Geometry check sheet. Reference: the model listing, model coordinates, mm. A direction names the side the tool comes from. Give positions to 0.01 mm unless a question says otherwise; leave off trailing zeros. Loops run counter-clockwise (first coordinate to the right, second up) from the corner with the lowest first, then second, coordinate; pieces in that order, holes last. Notation, with made-up numbers: (67.5, -9) -> (115.5, -9) arc R32 cw to (115.5, 22) -> close; hole circle Ø5 at (78.5, 77). An arc over 180 degrees is marked (long way). Answer as a JSON object with one key per item and string values.
from build123d import *

# Parameters (mm, degrees)
F1_DEPTH = 50.8
F2_W     = 38.1
F2_H     = 25.4
F3_DEPTH = 38.101
F5_D     = 12.7


with BuildPart() as f1:
    # F0 (on Front) → F1 (new body)
    with BuildSketch(Plane.XZ):
        Polygon((-41.500658, 3.663934), (-60.550658, 3.663934), (-60.550658, -34.436066), (28.349342, -34.436066), (28.349342, 3.663934), (15.649342, 3.663934), (15.649342, -17.219239), (-41.500658, -17.219239), align=None)
    extrude(amount=F1_DEPTH)

    # F2 (on face) → F3 (cut, through all)
    with BuildSketch(Plane(origin=(0, 0, -34.436066), x_dir=(1, 0, 0), z_dir=(0, 0, -1))):
        with Locations((9.299342, 38.1)):
            Rectangle(F2_W, F2_H)
    extrude(amount=-F3_DEPTH, mode=Mode.SUBTRACT)

    # F5 (through all)
    with Locations(Plane.XY.offset(-17.219239)):
        with Locations((-28.852955, -40.337186), (0, -9.016548)):
            Hole(F5_D / 2)


solid = f1.part
1) Depth check by flat-ended pin: P1, Ø10, axis at y = -36.5, z = -12, coming from the +X side; P2, Ø6, axis at x = -31.5, z = -12, coming from the -Y side; P3, Ø14.5, axis at x = -28.85, y = -40.34, coming from the +Z side; P4, Ø5, axis at y = -34, z = -25.5, coming from the +X side. Enter the tip coordinate at first touch or a pass-through.
Geometry check:
{"P1": "stops at x = -41.5", "P2": "passes through", "P3": "stops at z = -17.22", "P4": "stops at x = -9.75"}
2) Tool access check on faces 1 (the face through (-19, -19, -17.219)), 2 (the face through (28.349, -13, -16)), 3 (the face through (13, -25.4, -20)). Record the directions out of +Z, -Z, +X, -X, +Y, -Y that give a thin tool (end or side, any length) a straight path to the whole face; none if there is none.
Geometry check:
{"face 1": "+Z, +Y, -Y", "face 2": "+Z, -Z, +X, +Y, -Y", "face 3": "+Z, -Z, +X, -Y"}
3) Section check B-B on x = 0. Record the cut outline in (y, z).
Geometry check:
{"outline": "(-25.4, -34.44) -> (-15.37, -34.44) -> (-15.37, -17.22) -> (-25.4, -17.22) -> close; (-2.67, -34.44) -> (0, -34.44) -> (0, -17.22) -> (-2.67, -17.22) -> close"}
4) Material ranges on line 1 along X through (y, z) = (-16, -11.5); line 2 along Y through (x, z) = (0, -26.75); line 3 along Z through (x, y) = (-38, -17), recorded low to high. Write a range as from..to.
Geometry check:
{"line 1": "x = -60.55..-41.5, 15.65..28.35", "line 2": "y = -25.4..-15.37, -2.67..0", "line 3": "z = -34.44..-17.22"}
5) Section check D-D on y = -21.5. Record the cut outline in (x, z).
Geometry check:
{"outline": "(-60.55, -34.44) -> (28.35, -34.44) -> (28.35, 3.66) -> (15.65, 3.66) -> (15.65, -17.22) -> (-41.5, -17.22) -> (-41.5, 3.66) -> (-60.55, 3.66) -> close"}
6) Section check A-A on z = -1. Record the cut outline in (x, y), plus the area to 3 significant figures.
Geometry check:
{"outline": "(-60.55, -50.8) -> (-41.5, -50.8) -> (-41.5, 0) -> (-60.55, 0) -> close; (15.65, -25.4) -> (28.35, -25.4) -> (28.35, 0) -> (15.65, 0) -> close", "area": "1,290 mm2"}
7) Draft check along X on faces 4 (the face through (-51, -25, 3.664)), 5 (the face through (-9.751, -38, -26)), 6 (the face through (15.649, -13, -7)). Enter one of: pulls with the +X half, pulls with the -X half, needs draft (parallel to the pull), parting line crosses it, or undercut.
Geometry check:
{"face 4": "needs draft", "face 5": "pulls with the +X half", "face 6": "undercut"}
8) Section check C-C on z = -23.5. Record the cut outline in (x, y).
Geometry check:
{"outline": "(-60.55, -50.8) -> (-9.75, -50.8) -> (-9.75, -25.4) -> (28.35, -25.4) -> (28.35, 0) -> (-60.55, 0) -> close; hole circle Ø12.7 at (-28.85, -40.34); hole circle Ø12.7 at (0, -9.02)"}
